The listing builds one solid part. Answer for the finished solid, in the listing's coordinates (mm). Coordinates: 2 decimals unless noted, no trailing zeros. Order: outer loops, then holes, each group sorted by start corner. A loop starts at its lowest first (then second) coordinate and runs counter-clockwise, first axis right, second up. Notation, with made-up numbers: (-38, -37.75) - (6, -37.75) arc R29 ccw to (6, -5.75) - close; hole circle Ø8 at (-7, 46). An arc over 180 degrees is marked (long way). Use a Markdown table: item, result. Add a question column.
Item 1: Find the intervals of material crossed by line 1 along Y through (x, z) = (11, 9); line 2 along Y through (x, z) = (4, 8.25); line 3 along Z through (x, y) = (19.25, 4), in increasing order.
Item 2: The part is cut by section A-A, the plane y = 20. Give the vertices of the cut face in (x, z).
Item 3: A flat-ended cylindrical pin translates along its axis: P1, Ø2, axis at x = 16, y = 24, coming from the +Z side. Find the tip coordinate at first contact, or state that the pin passes through.
Item 4: The part is cut by section C-C, the plane y = 15.5. Give the vertices of the cut face in (x, z).
Item 5: The part is cut by section B-B, the plane x = 16.75. Give the vertices of the cut face in (y, z).
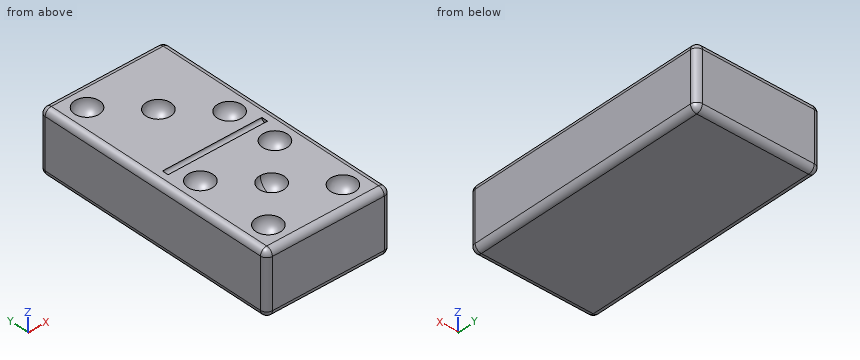
from build123d import *

# Parameters (mm, degrees)
CYLINDER_R               = 0.5
CYLINDER_DEPTH           = 16
ARRAY002_X_COUNT         = 3
ARRAY002_X_PITCH         = 8.485281
ARRAY001_X_COUNT         = 3
ARRAY001_X_PITCH         = 8.485281
ARRAY001_PLACEMENT_ANGLE = 90
ARRAY_X_COUNT            = 3
ARRAY_X_PITCH            = 8.485281
ARRAY_PLACEMENT_ANGLE    = 90
BOX_W                    = 20
BOX_H                    = 40
BOX_DEPTH                = 10
FILLET_R                 = 1


with BuildPart() as division:
    # Cylinder → Cylinder (new body)
    with BuildSketch(Plane(origin=(2, 20, 10), x_dir=(0, 0, -1), z_dir=(1, 0, 0))):
        Circle(CYLINDER_R)
    extrude(amount=CYLINDER_DEPTH)


with BuildPart() as array002:
    # Sphere002 → Sphere002 (revolve)
    with BuildSketch(Plane.XZ):
        with BuildLine():
            ThreePointArc((0, -2), (2, 0), (0, 2))
            Line((0, 2), (0, -2))
        make_face()
    revolve(axis=Axis((0, 0, 0), (0, 0, 1)))

    # Array002 X: Array002 ×3


with BuildPart() as array002_1:
    add(array002.part)
    with Locations(*[Vector(0.707107, 0.707107, 0) * (i * ARRAY002_X_PITCH) for i in range(1, ARRAY002_X_COUNT)]):
        add(array002.part)


with BuildPart() as cinco:
    # Sphere001 → Sphere001 (revolve)
    with BuildSketch(Plane.XZ):
        with BuildLine():
            ThreePointArc((0, -2), (2, 0), (0, 2))
            Line((0, 2), (0, -2))
        make_face()
    revolve(axis=Axis((0, 0, 0), (0, 0, 1)))

    # Array001 X: cinco ×3


with BuildPart() as cinco_1:
    add(cinco.part)
    with Locations(*[Vector(0.707107, 0.707107, 0) * (i * ARRAY001_X_PITCH) for i in range(1, ARRAY001_X_COUNT)]):
        add(cinco.part)


with BuildPart() as cinco_2:
    # Array001 placement: moved
    add(cinco_1.part.moved(Location((12, 0, 0))).rotate(Axis((12, 0, 0), (0, 0, 1)), ARRAY001_PLACEMENT_ANGLE))

    # Fusion: union Array002
    add(array002_1.part)


with BuildPart() as cinco_3:
    # Fusion placement: moved
    add(cinco_2.part.moved(Location((4, 4, 10))))


with BuildPart() as obj1:
    # Sphere → Sphere (revolve)
    with BuildSketch(Plane.XZ):
        with BuildLine():
            ThreePointArc((0, -2), (2, 0), (0, 2))
            Line((0, 2), (0, -2))
        make_face()
    revolve(axis=Axis((0, 0, 0), (0, 0, 1)))

    # Array X: obj1 ×3


with BuildPart() as obj1_1:
    add(obj1.part)
    with Locations(*[Vector(0.707107, 0.707107, 0) * (i * ARRAY_X_PITCH) for i in range(1, ARRAY_X_COUNT)]):
        add(obj1.part)


with BuildPart() as obj1_2:
    # Array placement: moved
    add(obj1_1.part.moved(Location((16, 24, 10))).rotate(Axis((16, 24, 10), (0, 0, 1)), ARRAY_PLACEMENT_ANGLE))

    # Fusion001: union cinco
    add(cinco_3.part)

    # Fusion002: union division
    add(division.part)


with BuildPart() as obj2:
    # Box → Box (new body)
    with BuildSketch(Plane.XY):
        with Locations((10, 20)):
            Rectangle(BOX_W, BOX_H)
    extrude(amount=BOX_DEPTH)

    # Fillet
    fillet_edges = [obj2.edges().sort_by_distance(p)[0] for p in [
        (0, 0, 5),
        (0, 20, 10),
        (0, 40, 5),
        (0, 20, 0),
        (20, 0, 5),
        (20, 20, 10),
        (20, 40, 5),
        (20, 20, 0),
        (10, 0, 0),
        (10, 0, 10),
        (10, 40, 0),
        (10, 40, 10),
    ]]
    fillet(fillet_edges, radius=FILLET_R)

    # Cut: cut obj1
    add(obj1_2.part, mode=Mode.SUBTRACT)


solid = obj2.part
Solution:
| question | item | result |
|---|---|---|
| 1 | line 1 | y = 0 to 8.59, 11.41 to 28.59, 31.41 to 40 |
| 1 | line 2 | y = 0 to 3.03, 4.97 to 15.03, 16.97 to 35.03, 36.97 to 40 |
| 1 | line 3 | z = 0.03 to 9.97 |
| 2 | outline | (0, 1) arc R1 ccw to (1, 0) - (19, 0) arc R1 ccw to (20, 1) - (20, 9) arc R1 ccw to (19, 10) - (18, 10) - (18, 9.5) - (2, 9.5) - (2, 10) - (1, 10) arc R1 ccw to (0, 9) - close |
| 3 | P1 | stops at z = 8.27 |
| 4 | outline | (0, 1) arc R1 ccw to (1, 0) - (19, 0) arc R1 ccw to (20, 1) - (20, 9) arc R1 ccw to (19, 10) - (17.94, 10) arc R1.94 cw to (14.06, 10) - (5.94, 10) arc R1.94 cw to (2.06, 10) - (1, 10) arc R1 ccw to (0, 9) - close |
| 5 | outline | (0, 1) arc R1 ccw to (1, 0) - (39, 0) arc R1 ccw to (40, 1) - (40, 9) arc R1 ccw to (39, 10) - (25.85, 10) arc R1.85 cw to (22.15, 10) - (20.5, 10) arc R0.5 cw to (19.5, 10) - (17.85, 10) arc R1.85 cw to (14.15, 10) - (5.85, 10) arc R1.85 cw to (2.15, 10) - (1, 10) arc R1 ccw to (0, 9) - close |
